Part print with two shaded views. Sizes in mm from the minimum x, y, z corner. A direction names the side the tool comes from. Coordinates: 2 decimals unless noted, no trailing zeros. Loops run counter-clockwise (first coordinate to the right, second up) from the corner with the lowest first, then second, coordinate; pieces in that order, holes last.
(1) Slice it at D-D (y = 3). Give the cut face in (x, z).
(2) Wall check: L1, parallel to X at y = 8.8, z = 4.5; L2, parallel to Y at x = 11.25, z = 12.5; L3, parallel to Z at x = 21.5, y = 5.5. Give the ranges that are in metal, low to high.
(3) Slice it at A-A (x = 11.5). Give the cut face in (y, z), and give its area (3 significant figures).
(4) Slice it at B-B (y = 8). Give the cut face in (x, z).
(5) Flat gauge pins, fed straight in: P1, Ø3, axis at x = 7.5, y = 3.5, coming from the -Z side; P2, Ø2.5, axis at y = 8.5, z = 16, coming from the +X side; P3, Ø1.5, axis at x = 9.5, z = 10, coming from the -Y side; P4, Ø3.5, axis at x = 11.5, z = 4.5, coming from the +Y side. Where does each tip first touch, or does it go through?
(6) Tool access for the marked faces 1, 2 and 3: list every direction of +Z, -Z, +X, -X, +Y, -Y with a clear straight run to the whole face (end or side of a thin tool).
(7) Slice it at C-C (z = 4.5). Give the cut face in (x, y).
(8) Two-plate mould, pull along Z, no slides. Class the marked faces 4, 5 and 6: pulls with the +Z half, pulls with the -Z half, needs draft (parallel to the pull), parting line crosses it, or undercut.
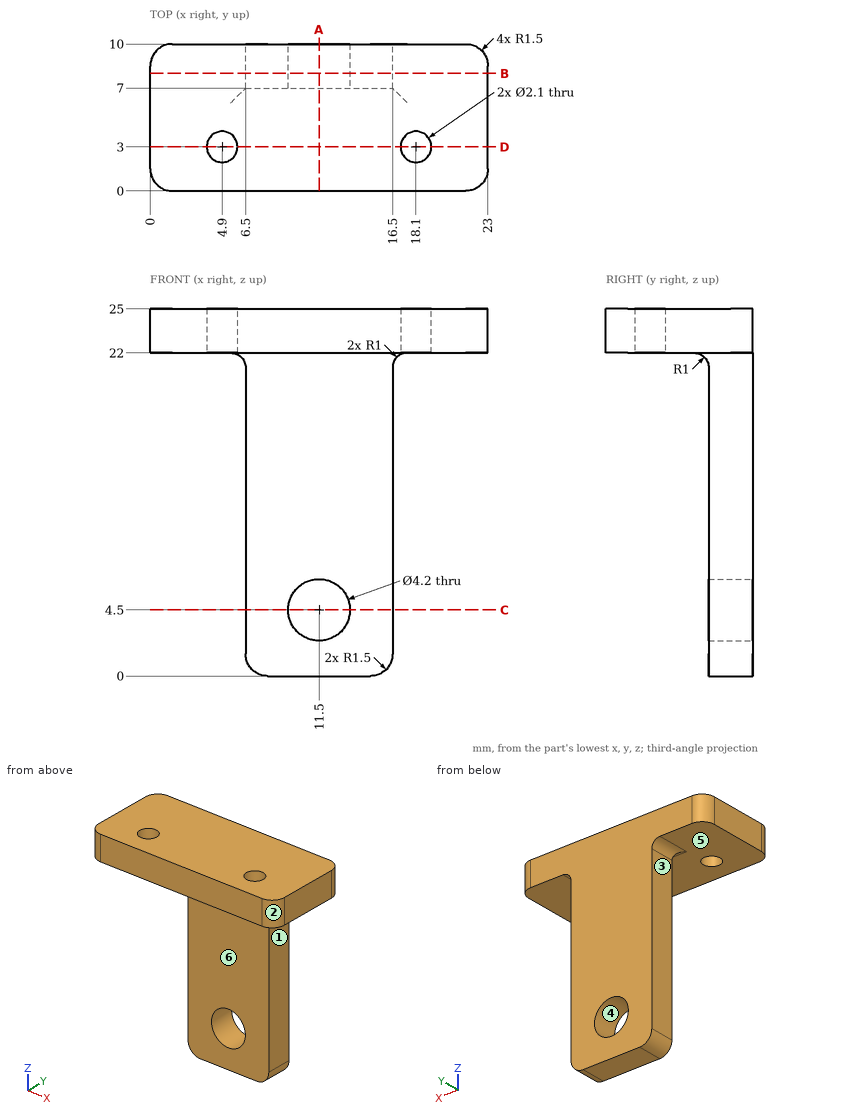
Response values:
1. outline: (0, 22) - (3.85, 22) - (3.85, 25) - (0, 25) - close; (5.95, 22) - (17.05, 22) - (17.05, 25) - (5.95, 25) - close; (19.15, 22) - (23, 22) - (23, 25) - (19.15, 25) - close
2. L1: x = 6.5 to 9.4, 13.6 to 16.5
2. L2: y = 7 to 10
2. L3: z = 22 to 25
3. outline: (0, 22) - (6, 22) arc R1 cw to (7, 21) - (7, 6.6) - (10, 6.6) - (10, 25) - (0, 25) - close; (7, 0) - (10, 0) - (10, 2.4) - (7, 2.4) - close
3. area: 83.6 mm2
4. outline: (0, 22) - (5.5, 22) arc R1 cw to (6.5, 21) - (6.5, 1.5) arc R1.5 ccw to (8, 0) - (15, 0) arc R1.5 ccw to (16.5, 1.5) - (16.5, 21) arc R1 cw to (17.5, 22) - (23, 22) - (23, 25) - (0, 25) - close; hole circle Ø4.2 at (11.5, 4.5)
5. P1: stops at z = 22
5. P2: stops at x = 16.5
5. P3: stops at y = 7
5. P4: passes through
6. face 1: -Z, +X, +Y, -Y
6. face 2: +Z, -Z, +X, -Y
6. face 3: -Z, -X, +Y, -Y
7. outline: (6.5, 7) - (9.4, 7) - (9.4, 10) - (6.5, 10) - close; (13.6, 7) - (16.5, 7) - (16.5, 10) - (13.6, 10) - close
8. face 4: undercut
8. face 5: pulls with the -Z half
8. face 6: needs draft
